Autodesk Inventor part; units mm, degrees
ref_plane "YZ Plane" through (0, 0, 0) normal (1, 0, 0) x (0, 1, 0)
ref_plane "XZ Plane" through (0, 0, 0) normal (0, 1, 0) x (-1, 0, 0)
ref_plane "XY Plane" through (0, 0, 0) normal (0, 0, 1) x (1, 0, 0)
sketch "Sketch1" plane through (0, 0, 0) normal (0, 0, 1) x (1, 0, 0)
  line L0 (146.05, -73.025) -> (-146.05, -73.025)
  line L1 (-146.05, -73.025) -> (-146.05, 73.025)
  line L2 (-146.05, 73.025) -> (146.05, 73.025)
  line L3 (146.05, 73.025) -> (146.05, -73.025)
  line L4 (146.05, -73.025) -> (-146.05, 73.025) construction
  line L5 (-146.05, -73.025) -> (146.05, 73.025) construction
  line L6 (-144.4625, 67.0179) -> (-144.4625, -67.0179)
  line L7 (-140.0429, -71.4375) -> (140.0429, -71.4375)
  line L8 (144.4625, -67.0179) -> (144.4625, 67.0179)
  line L9 (140.0429, 71.4375) -> (-140.0429, 71.4375)
  line L10 (-142.2527, -67.0179) -> (-142.2527, 67.0179)
  line L11 (-140.0429, 69.2277) -> (140.0429, 69.2277)
  line L12 (142.2527, 67.0179) -> (142.2527, -67.0179)
  line L13 (140.0429, -69.2277) -> (-140.0429, -69.2277)
  arc A0 (-142.2527, -67.0179) -> (-140.0429, -69.2277) centre (-140.0429, -67.0179) ccw
  arc A1 (140.0429, -69.2277) -> (142.2527, -67.0179) centre (140.0429, -67.0179) ccw
  arc A2 (142.2527, 67.0179) -> (140.0429, 69.2277) centre (140.0429, 67.0179) ccw
  arc A3 (-140.0429, 69.2277) -> (-142.2527, 67.0179) centre (-140.0429, 67.0179) ccw
  arc A4 (-144.4625, -67.0179) -> (-140.0429, -71.4375) centre (-140.0429, -67.0179) ccw
  arc A5 (140.0429, -71.4375) -> (144.4625, -67.0179) centre (140.0429, -67.0179) ccw
  arc A6 (144.4625, 67.0179) -> (140.0429, 71.4375) centre (140.0429, 67.0179) ccw
  arc A7 (-140.0429, 71.4375) -> (-144.4625, 67.0179) centre (-140.0429, 67.0179) ccw
  point P0 (0, 0)
  dimension "d0" = 292.1
  dimension "d1" = 146.05
  dimension "d2" = 1.5875
  dimension "d3" = 2.2098
  dimension "d4" = 2.2098
  dimension "d5" = 4.4196
extrude "Extrusion1" add sketch "Sketch1" along normal blind 1.1684 contours A7 L9 A6 L8 A5 L7 A4 L6
fillet "Fillet1" radius 0.5 32 edges at (-141.6055, 68.5805, 1.1684) (0, 69.2277, 1.1684) (141.6055, 68.5805, 1.1684) (142.2527, 0, 1.1684) (141.6055, -68.5805, 1.1684) (0, -69.2277, 1.1684) (-141.6055, -68.5805, 1.1684) (-142.2527, 0, 1.1684) (-141.6055, 68.5805, 0) (-142.2527, 0, 0) (-141.6055, -68.5805, 0) (0, -69.2277, 0) (141.6055, -68.5805, 0) (142.2527, 0, 0) (141.6055, 68.5805, 0) (0, 69.2277, 0) (-144.4625, 0, 1.1684) (-143.168, -70.143, 1.1684) (0, -71.4375, 1.1684) (143.168, -70.143, 1.1684) (144.4625, 0, 1.1684) (143.168, 70.143, 1.1684) (0, 71.4375, 1.1684) (-143.168, 70.143, 1.1684) (-144.4625, 0, 0) (-143.168, 70.143, 0) (0, 71.4375, 0) (143.168, 70.143, 0) (144.4625, 0, 0) (143.168, -70.143, 0) (0, -71.4375, 0) (-143.168, -70.143, 0)
equation "\"d0\" = depth + 2 * frameAcrylicThickness"
equation "\"d1\" = width + 2 * frameAcrylicThickness"
equation "\"frameAcrylicThickness\" = 9.525"
equation "\"width\" = 127"
equation "\"depth\" = 273.05"
equation "\"internalAcrylicThickness\" = 6.35"
equation "\"height\" = 127"
equation "\"mirrorAngle\" = 5deg"
equation "\"detectorWidth\" = 52"
equation "\"detectorHeight\" = 52"
equation "\"mirrorThickness\" = 3.175"
equation "\"fresnelThickness\" = 0.1"
equation "\"focalLength\" = 76.2"
equation "\"ior\" = 1.49"
equation "\"centerThickness\" = 1.524"
equation "\"fresnelAngle\" = 90deg"
equation "\"fresnelEffectiveDiameter\" = 152.4"
equation "\"oRingWidth\" = 1.5875"
equation "\"sensorHolderDepth\" = 19.05"
equation "\"aerogelClearence\" = 3.175"
equation "\"backplanePCBHeight\" = 76.2"
equation "\"backplanePCBWidth\" = 76.2"
equation "\"backplaneHoleOffsett\" = 6.35"
equation "\"backplanePostionOffsett\" = 12.7"
equation "\"moduleSlotClearence\" = 0.79375"
properties part number "topORing" material "Rubber"
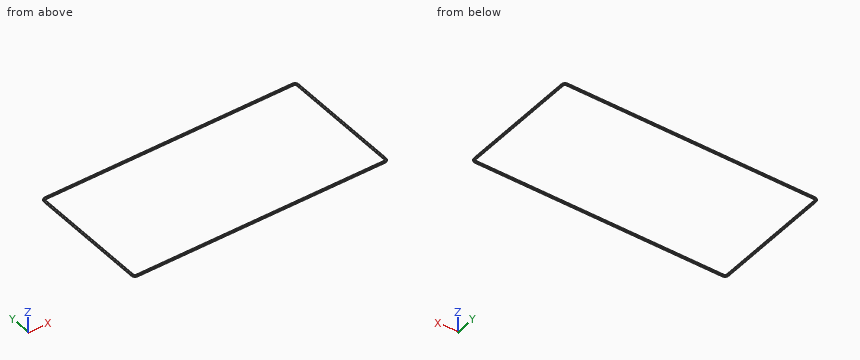
Can you work these out from the model? Positions are in its coordinate system, mm. Coordinates: 2 decimals unless noted, no trailing zeros. Order: outer loops, then holes, each group sorted by start corner. A loop starts at its lowest first (then second) coordinate and runs counter-clockwise, first axis right, second up. Notation, with made-up numbers: (19.25, -13.75) -> (58.25, -13.75) arc R19 ccw to (58.25, 19.25) -> close; hole circle Ø8 at (69.5, 12). An arc over 180 degrees is marked (long way). Use one line per item in the form item = value.
Q1. Imagine slicing it at A-A, the plane y = -52. List the corners of the cut face in (x, z) for me.
From the geometry:
outline = (-144.46, 0.5) arc R0.5 ccw to (-143.96, 0) -> (-142.75, 0) arc R0.5 ccw to (-142.25, 0.5) -> (-142.25, 0.67) arc R0.5 ccw to (-142.75, 1.17) -> (-143.96, 1.17) arc R0.5 ccw to (-144.46, 0.67) -> close; (142.25, 0.5) arc R0.5 ccw to (142.75, 0) -> (143.96, 0) arc R0.5 ccw to (144.46, 0.5) -> (144.46, 0.67) arc R0.5 ccw to (143.96, 1.17) -> (142.75, 1.17) arc R0.5 ccw to (142.25, 0.67) -> close
Q2. I need wall thicknesses on L1, parallel to Y at x = 50.5, z = 0.3; L2, parallel to X at y = 4, z = 0.75; L3, parallel to X at y = -21, z = 0.8. Which ranges of each line are inside material? Lowest first, please.
From the geometry:
L1 = -71.4 to -69.27, 69.27 to 71.4
L2 = -144.46 to -142.26, 142.26 to 144.46
L3 = -144.44 to -142.27, 142.27 to 144.44
Q3. Imagine slicing it at B-B, the plane x = -97. List the corners of the cut face in (y, z) for me, then the cut area to 3 significant figures.
From the geometry:
outline = (-71.44, 0.5) arc R0.5 ccw to (-70.94, 0) -> (-69.73, 0) arc R0.5 ccw to (-69.23, 0.5) -> (-69.23, 0.67) arc R0.5 ccw to (-69.73, 1.17) -> (-70.94, 1.17) arc R0.5 ccw to (-71.44, 0.67) -> close; (69.23, 0.5) arc R0.5 ccw to (69.73, 0) -> (70.94, 0) arc R0.5 ccw to (71.44, 0.5) -> (71.44, 0.67) arc R0.5 ccw to (70.94, 1.17) -> (69.73, 1.17) arc R0.5 ccw to (69.23, 0.67) -> close
area = 4.73 mm²
Q4. Imagine slicing it at C-C, the plane z = 0.2. List the corners of the cut face in (x, y) for me, then the cut area to 3 significant figures.
From the geometry:
outline = (-144.36, -67.02) arc R4.32 ccw to (-140.04, -71.34) -> (140.04, -71.34) arc R4.32 ccw to (144.36, -67.02) -> (144.36, 67.02) arc R4.32 ccw to (140.04, 71.34) -> (-140.04, 71.34) arc R4.32 ccw to (-144.36, 67.02) -> close; hole (-142.35, -67.02) arc R2.31 ccw to (-140.04, -69.33) -> (140.04, -69.33) arc R2.31 ccw to (142.35, -67.02) -> (142.35, 67.02) arc R2.31 ccw to (140.04, 69.33) -> (-140.04, 69.33) arc R2.31 ccw to (-142.35, 67.02) -> close
area = 1,710 mm²
